Work out the finished part from the listing and answer in its coordinate system (mm). A direction names the side the tool comes from. Give positions to 0.01 mm unless a question says otherwise; leave off trailing zeros. Write each loop counter-clockwise with the first axis right and the second up, starting at its lowest first coordinate (ties: lowest second). Pieces come first, ordered by that corner, then holes.
1) Straight lines are drawn through the part: probe 1 along Y at (x, z) = (-4.25, 7); probe 2 along Y at (x, z) = (3, -3.25); probe 3 along X at (y, z) = (10, 0.25). For each, find the intervals that lie inside material, in ascending order.
2) Find section D-D (y = 26.5). Determine the outline of the cut face in (x, z) (3 decimals), plus the area to 3 significant figures.
3) A tool of negligible diameter and unlimited length cuts with its end or side. For faces 1 (the face through (0, 27, 2.325)), 2 (the face through (-10.6, -6.3, -2.8)), 3 (the face through (-6, 12.2, 6)), 4 (the face through (0, 32.2, 0)), 5 (the face through (-3, -3.1, -3.3)), from which of +Z, -Z, +X, -X, +Y, -Y can it reach the whole face along a straight path? Write none if from no direction.
4) Given pin 1 Ø6 at (x, z) = (10, -4.5) entering from -Y; pin 2 Ø1.5 at (y, z) = (-0.5, -2.5) entering from +X; pin 3 Ø5 at (x, y) = (-6.5, 5) entering from -Z, each flat-ended and moving along its own axis, determine where each tip first touches the part or whether it passes through.
5) Determine the mould class of faces 6 (the face through (-10.13, -3.11, -2.78)), 7 (the face through (2.9, 18.26, -3.78)), 8 (the face through (10, 16.2, 0)), 9 (the face through (-10.13, -3.11, 2.91)) for opening direction Z: pulls with the +Z half, pulls with the -Z half, needs draft (parallel to the pull), parting line crosses it, or undercut.
6) Find section C-C (y = 4). Determine the outline of the cut face in (x, z).
```python
from build123d import *

# Parameters (mm, degrees)
CUT_EXTRUDE1_DEPTH  = 10
SKETCH6_R           = 1.5
BOSS_EXTRUDE3_DEPTH = 4
SKETCH7_R           = 0.5
BOSS_EXTRUDE4_DEPTH = 6.3


with BuildPart() as part:
    # Sketch1 → Revolve1 (revolve)
    with BuildSketch(Plane(origin=(0, 0, 0), x_dir=(0, 0, -1), z_dir=(1, 0, 0))):
        Polygon((0, 0), (-13, 0), (-13, 12.2), (-7.95, 12.2), (-7.95, 14.2), (-4.7625, 14.2), (-4.7625, 22.2), (-3.175, 22.2), (-3.175, 32.2), (0, 32.2), align=None)
    revolve(axis=Axis((0, 0, 0), (0, -1, 0)))

    # Sketch3 → Cut-Extrude1 (cut)
    with BuildSketch(Plane(origin=(0, 32.2, 0), x_dir=(1, 0, 0), z_dir=(0, 1, 0))):
        with BuildLine():
            Line((-2.162174831, -2.325), (2.162174831, -2.325))
            ThreePointArc((2.162174831, -2.325), (0, -3.175), (-2.162174831, -2.325))
        make_face()
    extrude(amount=-CUT_EXTRUDE1_DEPTH, mode=Mode.SUBTRACT)

    # Sketch6 → Boss-Extrude3 (add)
    with BuildSketch(Plane(origin=(0, 12.2, 0), x_dir=(1, 0, 0), z_dir=(0, 1, 0))):
        with Locations(Location((9.5, 0, 0), (0, 0, 270))):
            Circle(SKETCH6_R)
    extrude(amount=BOSS_EXTRUDE3_DEPTH)

    # Sketch7 → Boss-Extrude4 (add)
    with BuildSketch(Plane.XZ):
        with Locations(Location((-2.847009496, -10.625184089, 0), (0, 0, 270))):
            Circle(SKETCH7_R)
        with Locations(Location((-7.778174593, -7.778174593, 0), (0, 0, 270))):
            Circle(SKETCH7_R)
        with Locations(Location((-2.828427125, -2.828427125, 0), (0, 0, 270))):
            Circle(SKETCH7_R)
        with Locations(Location((-10.625184089, -2.847009496, 0), (0, 0, 270))):
            Circle(SKETCH7_R)
        with Locations(Location((-10.625184089, 2.847009496, 0), (0, 0, 270))):
            Circle(SKETCH7_R)
    extrude(amount=BOSS_EXTRUDE4_DEPTH)


solid = part.part
```
Results:
1. probe 1: y = 0 to 12.2
1. probe 2: y = 0 to 22.2
1. probe 3: x = -13 to 13
2. outline: (-2.162, 2.325) arc R3.175 ccw (long way) to (2.162, 2.325) - close
2. area: 29.1 mm2
3. face 1: +Z, +X, -X, +Y
3. face 2: +Z, -Z, +X, -X, -Y
3. face 3: +Y
3. face 4: +Z, -Z, +X, -X, +Y
3. face 5: -Y
4. pin 1: stops at y = 0
4. pin 2: stops at x = 12.85
4. pin 3: stops at z = -12.37
5. face 6: undercut
5. face 7: parting line crosses it
5. face 8: needs draft
5. face 9: undercut
6. outline: circle Ø26 at (0, 0)
